Build history of the part. All positions in model axes, mm. Face numbers are marked on the shaded views. A direction names the side the tool comes from. Give positions to 0.01 mm unless a question says otherwise; leave off trailing zeros. Loops run counter-clockwise (first coordinate to the right, second up) from the corner with the lowest first, then second, coordinate; pieces in that order, holes last. Notation, with made-up numbers: (41, 36.5) - (83, 36.5) arc R35 ccw to (83, 70.5) - close; hole circle Ø3 at (12, 71). An arc over 180 degrees is marked (long way). Return JSON: item names as keys, results as strings. Group by question number.
1) Drill centre lines: probe 1 along X at (y, z) = (36.6, 17.4); probe 2 along X at (y, z) = (35.5, 18.75); probe 3 along Y at (x, z) = (-17.5, 24). Where is each one in solid material? Low to high. Write a range as from..to.
2) Drop flat-ended pins along their axis: pin 1 (4 mm diameter, centred on x = -18, z = 14.5, fed in from +Y); pin 2 (10 mm diameter, centred on y = 29.5, z = 8, fed in from +X); pin 3 (4 mm diameter, centred on x = 8, y = 28.5, fed in from +Z). Give the stop position or say it passes through.
3) Mould opens along Z. For the marked faces 4, 5 and 6 say: released by +Z, released by -Z, zero draft, split by the parting line, or undercut.
4) 3-axis set-ups, long thin cutter, end or side, ignore diameter. For the marked faces 1, 2 and 3: which of +Z, -Z, +X, -X, +Y, -Y reach the whole face in a straight line?
5) Slice it at B-B (y = 29.75). List the corners of the cut face in (x, z).
6) Slice it at A-A (z = 21.25). List the corners of the cut face in (x, y).
7) Slice it at D-D (y = 52). List the corners of the cut face in (x, z), and give its area (3 significant figures).
8) Slice it at C-C (z = 17.4). List the corners of the cut face in (x, y), and give its area (3 significant figures).
```python
from build123d import *

# Parameters (mm, degrees)
PAD026_DEPTH            = 34
SKETCH034_R             = 0.9
POCKET006_DEPTH         = 12.001
SKETCH036_W             = 13
SKETCH036_H             = 23.2
POCKET007_DEPTH         = 12.001
SKETCH037_R             = 1.4
PAD027_DEPTH            = 1.6
SKETCH038_R             = 1.4
PAD028_DEPTH            = 1.6
SKETCH039_W             = 10
SKETCH039_H             = 7
SKETCH039_R             = 0.9
PAD029_DEPTH            = 5
CHAMFER002_SIZE         = 1.6
BODY006_PLACEMENT_ANGLE = 90


with BuildPart() as part:
    # Sketch035 → Pad026 (new body)
    with BuildSketch(Plane.XZ):
        Polygon((-12, 1.6), (-9, 1.6), (-4, 6.6), (-4, 22.2), (0, 22.2), (0, 6.6), (4, 1.6), (4, 0), (-3.601763, 0), (-12, 0), align=None)
    extrude(amount=PAD026_DEPTH)

    # Sketch034 → Pocket006 (cut, through all)
    with BuildSketch(Plane(origin=(0, 0, 0), x_dir=(0, 0, 1), z_dir=(1, 0, 0))):
        with Locations((13.4, 30.8)):
            Circle(SKETCH034_R)
        with Locations((13.4, 3.6)):
            Circle(SKETCH034_R)
    extrude(amount=-POCKET006_DEPTH, mode=Mode.SUBTRACT)

    # Sketch036 (on DatumPlane) → Pocket007 (cut, through all)
    with BuildSketch(Plane(origin=(0, 0, 0), x_dir=(0, 0, 1), z_dir=(1, 0, 0))):
        with Locations((13.4, 17.2)):
            Rectangle(SKETCH036_W, SKETCH036_H)
    extrude(amount=-POCKET007_DEPTH, mode=Mode.SUBTRACT)

    # Sketch037 → Pad027 (join)
    with BuildSketch(Plane.XY):
        with BuildLine():
            ThreePointArc((-17.5, 0), (-19.888457, -1.184712), (-20.390493, -3.803152))
            Line((-12, -34), (-20.390493, -3.803152))
            Line((-11.5, -34), (-12, -34))
            Line((-11.5, 0), (-11.5, -34))
            Line((-11.5, 0), (-17.5, 0))
        make_face()
        with Locations((-17.5, -3)):
            Circle(SKETCH037_R, mode=Mode.SUBTRACT)
    extrude(amount=PAD027_DEPTH)

    # Sketch038 → Pad028 (join)
    with BuildSketch(Plane.XY):
        with BuildLine():
            ThreePointArc((6, -34), (8.894987, -31.786799), (7.518515, -28.412702))
            Line((0, -24), (7.518515, -28.412702))
            Line((0, -34), (0, -24))
            Line((0, -34), (6, -34))
        make_face()
        with Locations((6, -31)):
            Circle(SKETCH038_R, mode=Mode.SUBTRACT)
        with BuildLine():
            ThreePointArc((7.518515, -5.587298), (8.894988, -2.213208), (6.000014, 0))
            Line((0, 0), (6.000014, 0))
            Line((0, 0), (0, -10))
            Line((0, -10), (7.518515, -5.587298))
        make_face()
        with Locations((6, -3)):
            Circle(SKETCH038_R, mode=Mode.SUBTRACT)
    extrude(amount=PAD028_DEPTH)

    # Sketch039 (on Face3 of Pad028) → Pad029 (join)
    with BuildSketch(Plane(origin=(0, 0, 0), x_dir=(0, 0, 1), z_dir=(1, 0, 0))):
        with Locations((13.4, 32.3)):
            Rectangle(SKETCH039_W, SKETCH039_H)
        with Locations((13.4, 30.8)):
            Circle(SKETCH039_R, mode=Mode.SUBTRACT)
        with Locations((13.4, 2.1)):
            Rectangle(SKETCH039_W, SKETCH039_H)
        with Locations((13.4, 3.6)):
            Circle(SKETCH039_R, mode=Mode.SUBTRACT)
    extrude(amount=-PAD029_DEPTH)

    # Chamfer002
    chamfer002_edges = [part.edges().sort_by_distance(p)[0] for p in [
        (-2, 0, 22.2),
        (-2, -34, 22.2),
    ]]
    chamfer(chamfer002_edges, length=CHAMFER002_SIZE)


with BuildPart() as part_1:
    # Body006 placement: moved
    add(part.part.moved(Location((12.020815, 35.221825, 4))).rotate(Axis((12.020815, 35.221825, 4), (0, 0, -1)), BODY006_PLACEMENT_ANGLE))


solid = part_1.part
```
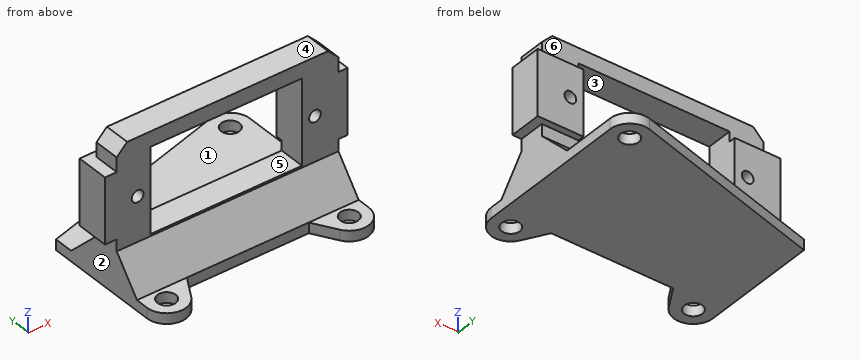
Results:
{
 "1": {"probe 1": "-23.78..-19.68, -17.88..-16.78, 6.42..7.52, 9.32..13.42", "probe 2": "-23.78..-16.78, 6.42..13.42", "probe 3": "35.22..39.22"},
 "2": {"pin 1": "y = 40.22", "pin 2": "x = 12.02", "pin 3": "z = 5.6"},
 "3": {"face 4": "released by +Z", "face 5": "undercut", "face 6": "zero draft"},
 "4": {"face 1": "+Z, +X, -X, +Y", "face 2": "-Z, -X, +Y, -Y", "face 3": "+Y, -Y"},
 "5": {"outline": "(-21.98, 4) - (-20.28, 4) - (-20.28, 5.6) - (-21.98, 5.6) - close; (-17.68, 4) - (-15.19, 4) - (-15.19, 5.6) - (-17.68, 5.6) - close; (5.23, 4) - (7.72, 4) - (7.72, 5.6) - (5.23, 5.6) - close; (10.32, 4) - (12.02, 4) - (12.02, 5.6) - (10.32, 5.6) - close"},
 "6": {"outline": "(-23.78, 35.22) - (-16.78, 35.22) - (-16.78, 40.22) - (-23.78, 40.22) - close; (6.42, 35.22) - (13.42, 35.22) - (13.42, 40.22) - (6.42, 40.22) - close"},
 "7": {"outline": "(-4.78, 4) - (7.82, 4) - (7.82, 5.6) - (-4.78, 5.6) - close; (10.22, 4) - (12.02, 4) - (12.02, 5.6) - (10.22, 5.6) - close", "area": "23.0 mm2"},
 "8": {"outline": "(-23.78, 35.22) - (-19.68, 35.22) - (-19.68, 40.22) - (-23.78, 40.22) - close; (-17.88, 35.22) - (-16.78, 35.22) - (-16.78, 40.22) - (-17.88, 40.22) - close; (6.42, 35.22) - (7.52, 35.22) - (7.52, 40.22) - (6.42, 40.22) - close; (9.32, 35.22) - (13.42, 35.22) - (13.42, 40.22) - (9.32, 40.22) - close", "area": "52.0 mm2"}
}
